Read the model definition and answer for the solid it produces. Units are mm, in the model's axes. A direction names the side the tool comes from. Round coordinates to 2 decimals unless told otherwise and drop trailing zeros. Write each loop counter-clockwise with the first axis right and the second up, starting at its lowest first coordinate (ties: lowest second). Pieces come first, ordered by that corner, then holes.
from build123d import *

# Parameters (mm, degrees)
F1_DEPTH  = 48
F2_R      = 5.5
F3_DEPTH  = 50.001
F4_R      = 6.5
F5_DEPTH  = 20
F6_R      = 8.5
F7_DEPTH  = 30.85
F8_R      = 1.21
F9_DEPTH  = 50.001
F10_R     = 10
F11_DEPTH = 10
F12_R     = 3
F13_DEPTH = 20


with BuildPart() as f1:
    # F0 (on Front) → F1 (new body)
    with BuildSketch(Plane.XZ):
        Polygon((-140, 0), (0, 0), (0, 50), (-63.5, 50), (-76.5, 50), (-140, 50), align=None)
    extrude(amount=F1_DEPTH)

    # F2 (on face) → F3 (cut, through all)
    with BuildSketch(Plane.XY.offset(50)):
        with Locations((-123.75, -33.112)):
            Circle(F2_R)
        with Locations((-16.25, -33.112)):
            Circle(F2_R)
    extrude(amount=-F3_DEPTH, mode=Mode.SUBTRACT)

    # F4 (on face) → F5 (cut)
    with BuildSketch(Plane.XZ.offset(48)):
        with Locations((-70, 50)):
            Circle(F4_R)
    extrude(amount=-F5_DEPTH, mode=Mode.SUBTRACT)

    # F6 (on face) → F7 (cut)
    with BuildSketch(Plane(origin=(0, 0, 0), x_dir=(-1, 0, 0), z_dir=(0, 1, 0))):
        with Locations((70, 50)):
            Circle(F6_R)
    extrude(amount=-F7_DEPTH, mode=Mode.SUBTRACT)

    # F8 (on face) → F9 (cut, through all)
    with BuildSketch(Plane.XY.offset(50)):
        with Locations((-70, -33.112198)):
            Circle(F8_R)
    extrude(amount=-F9_DEPTH, mode=Mode.SUBTRACT)

    # F10 (on face) → F11 (cut)
    with BuildSketch(Plane(origin=(0, 0, 0), x_dir=(1, 0, 0), z_dir=(0, 0, -1))):
        with Locations((-70, 33.112198)):
            Circle(F10_R)
    extrude(amount=-F11_DEPTH, mode=Mode.SUBTRACT)

    # F12 (on face) → F13 (cut)
    with BuildSketch(Plane(origin=(0, 0, 10), x_dir=(1, 0, 0), z_dir=(0, 0, -1))):
        with Locations((-70, 33.112198)):
            Circle(F12_R)
    extrude(amount=-F13_DEPTH, mode=Mode.SUBTRACT)


solid = f1.part
Q1. Section A-A (x = -16.25) is taken. Determine the outline of the cut face in (y, z).
Verdict:
outline: (-48, 0) - (-38.61, 0) - (-38.61, 50) - (-48, 50) - close; (-27.61, 0) - (0, 0) - (0, 50) - (-27.61, 50) - close
Q2. Flat-ended cylindrical pins translate along their axes: pin 1 Ø6 at (x, y) = (-74.5, -36.5) entering from -Z; pin 2 Ø1.8 at (x, y) = (-71, -34) entering from -Z; pin 3 Ø9.5 at (x, z) = (-69, 46.5) entering from +Y. Find the tip coordinate at first contact, or state that the pin passes through.
Verdict:
pin 1: stops at z = 10
pin 2: stops at z = 30
pin 3: stops at y = -30.85
Q3. Determine the mould class of faces 4 (the cylindrical face through (-70.89, -32.29, 36.9)), 5 (the flat face through (-69, -32, 30)), 6 (the flat face through (-140, -24, 25)), 7 (the flat face through (-69, -30.85, 43)) for opening direction Y: pulls with the +Y half, pulls with the -Y half, needs draft (parallel to the pull), parting line crosses it, or undercut.
Verdict:
face 4: undercut
face 5: undercut
face 6: needs draft
face 7: pulls with the +Y half
Q4. Section B-B (z = 19) is taken. Determine the outline of the cut face in (x, y), then the cut area to 3 significant figures.
Verdict:
outline: (-140, -48) - (0, -48) - (0, 0) - (-140, 0) - close; hole circle Ø11 at (-123.75, -33.11); hole circle Ø6 at (-70, -33.11); hole circle Ø11 at (-16.25, -33.11)
area: 6,500 mm2
Q5. Which of the six approach directions +Z, -Z, +X, -X, +Y, -Y give full straight-line access (tool end or side, diameter ignored) to faces 1 (the flat face through (-71, 0, 25)), 2 (the flat face through (-67.9, -35.5, 10)), 3 (the cylindrical face through (-69.813, -15.209, 41.502))?
Verdict:
face 1: +Z, -Z, +X, -X, +Y
face 2: -Z
face 3: +Z, +Y
Q6. Section C-C (y = -17) is taken. Determine the outline of the cut face in (x, z).
Verdict:
outline: (-140, 0) - (0, 0) - (0, 50) - (-61.5, 50) arc R8.5 cw to (-78.5, 50) - (-140, 50) - close
Q7. Straight lines are drawn through the part: probe 1 along Y at (x, z) = (-16.25, 27); probe 2 along Y at (x, z) = (-70, 6.25); probe 3 along X at (y, z) = (-28.5, 43.5). For each, find the intervals that lie inside material, in ascending order.
Verdict:
probe 1: y = -48 to -38.61, -27.61 to 0
probe 2: y = -48 to -43.11, -23.11 to 0
probe 3: x = -140 to -126.75, -120.75 to -75.48, -64.52 to -19.25, -13.25 to 0
Q8. Section D-D (x = -126.5) is taken. Determine the outline of the cut face in (y, z), then the cut area to 3 significant figures.
Verdict:
outline: (-48, 0) - (-37.88, 0) - (-37.88, 50) - (-48, 50) - close; (-28.35, 0) - (0, 0) - (0, 50) - (-28.35, 50) - close
area: 1,920 mm2
